from build123d import *

# Parameters (mm, degrees)
F0_R     = 4.05
F1_DEPTH = 20
F2_DEPTH = 17
F3_R     = 3
F4_R     = 4.05
F5_DEPTH = 219.9
F6_START = 103.2
F6_DEPTH = 43.7
F7_DEPTH = 8


with BuildPart() as f1:
    # F0 (on Top) → F1 (new body)
    with BuildSketch(Plane.XY):
        with BuildLine():
            Line((80, 54.9215728753), (80, 47.75))
            Line((80, 47.75), (100, 20))
            Line((100, 20), (100, 0))
            Line((100, 0), (100, -20))
            Line((100, -20), (80, -47.75))
            Line((80, -47.75), (80, -63.952777299))
            Line((80, -63.952777299), (92, -65))
            Line((92, -65), (112, -64.6363035163))
            Line((112, -64.6363035163), (112, 0))
            Line((112, 0), (112, 64.1046091914))
            Line((112, 64.1046091914), (81.7398235416, 64.1046091914))
            Line((81.7398235416, 64.1046091914), (80, 63.952777299))
            Line((80, 63.952777299), (80, 60.5784271247))
            ThreePointArc((80, 60.5784271247), (80.4926940638, 60.706795679), (81, 60.75))
            Line((81, 60.75), (89, 60.75))
            Line((89, 60.75), (95, 60.75))
            Line((95, 60.75), (105, 60.75))
            ThreePointArc((105, 60.75), (107.1213203436, 59.8713203436), (108, 57.75))
            ThreePointArc((108, 57.75), (107.1213203436, 55.6286796564), (105, 54.75))
            Line((105, 54.75), (95, 54.75))
            Line((95, 54.75), (89, 54.75))
            Line((89, 54.75), (81, 54.75))
            ThreePointArc((81, 54.75), (80.4926940638, 54.793204321), (80, 54.9215728753))
        make_face()
        with Locations((92, -47.75)):
            Circle(F0_R, mode=Mode.SUBTRACT)
        with Locations((92, 47.75)):
            Circle(F0_R, mode=Mode.SUBTRACT)
        Polygon((80, -63.952777299), (80, -47.75), (74.5151937008, -55.3601687402), (74.5151937008, -63.4741261601), align=None)
        with BuildLine():
            Line((74.5151937008, 55.3601687402), (80, 47.75))
            Line((80, 47.75), (80, 54.9215728753))
            ThreePointArc((80, 54.9215728753), (78, 57.75), (80, 60.5784271247))
            Line((80, 60.5784271247), (80, 63.952777299))
            Line((80, 63.952777299), (74.5151937008, 63.4741261601))
            Line((74.5151937008, 63.4741261601), (74.5151937008, 55.3601687402))
        make_face()
    extrude(amount=F1_DEPTH)

    # F0 (on Top) → F2 (join)
    with BuildSketch(Plane.XY):
        with BuildLine():
            ThreePointArc((105, 60.75), (102, 57.75), (105, 54.75))
            ThreePointArc((105, 54.75), (107.1213203436, 55.6286796564), (108, 57.75))
            ThreePointArc((108, 57.75), (107.1213203436, 59.8713203436), (105, 60.75))
        make_face()
        with BuildLine():
            Line((80, 60.5784271247), (80, 54.9215728753))
            ThreePointArc((80, 54.9215728753), (80.4926940638, 54.793204321), (81, 54.75))
            ThreePointArc((81, 54.75), (83.1213203436, 55.6286796564), (84, 57.75))
            ThreePointArc((84, 57.75), (83.1213203436, 59.8713203436), (81, 60.75))
            ThreePointArc((81, 60.75), (80.4926940638, 60.706795679), (80, 60.5784271247))
        make_face()
        with BuildLine():
            ThreePointArc((80, 60.5784271247), (78, 57.75), (80, 54.9215728753))
            Line((80, 54.9215728753), (80, 60.5784271247))
        make_face()
        with BuildLine():
            ThreePointArc((84, 57.75), (83.1213203436, 55.6286796564), (81, 54.75))
            Line((81, 54.75), (89, 54.75))
            ThreePointArc((89, 54.75), (86, 57.75), (89, 60.75))
            Line((89, 60.75), (81, 60.75))
            ThreePointArc((81, 60.75), (83.1213203436, 59.8713203436), (84, 57.75))
        make_face()
        with BuildLine():
            ThreePointArc((98, 57.75), (97.1213203436, 55.6286796564), (95, 54.75))
            Line((95, 54.75), (105, 54.75))
            ThreePointArc((105, 54.75), (102, 57.75), (105, 60.75))
            Line((105, 60.75), (95, 60.75))
            ThreePointArc((95, 60.75), (97.1213203436, 59.8713203436), (98, 57.75))
        make_face()
    extrude(amount=F2_DEPTH)

    # F3
    f3_edges = [f1.edges().sort_by_distance(p)[0] for p in [
        (74.515194, -55.360169, 10),
        (74.515194, -63.474126, 10),
        (100, -20, 10),
        (100, 20, 10),
        (74.515194, 55.360169, 10),
        (74.515194, 63.474126, 10),
    ]]
    fillet(f3_edges, radius=F3_R)

    # F4 (on Right) → F5 (cut)
    with BuildSketch(Plane.YZ):
        with Locations((0, 10)):
            Circle(F4_R)
    extrude(amount=F5_DEPTH, mode=Mode.SUBTRACT)

    # F4 (on Right) → F6 (cut)
    with BuildSketch(Plane.YZ.offset(F6_START)):
        Polygon((-3.7527767497, 3.5), (3.7527767497, 3.5), (7.5055534995, 10), (3.7527767497, 16.5), (-3.7527767497, 16.5), (-7.5055534995, 10), align=None)
        with Locations((0, 10)):
            Circle(F4_R, mode=Mode.SUBTRACT)
    extrude(amount=F6_DEPTH, mode=Mode.SUBTRACT)

    # F0 (on Top) → F7 (join)
    with BuildSketch(Plane.XY):
        with BuildLine():
            ThreePointArc((89, 60.75), (86, 57.75), (89, 54.75))
            ThreePointArc((89, 54.75), (91.1213203436, 55.6286796564), (92, 57.75))
            ThreePointArc((92, 57.75), (91.1213203436, 59.8713203436), (89, 60.75))
        make_face()
        with BuildLine():
            Line((95, 60.75), (89, 60.75))
            ThreePointArc((89, 60.75), (91.1213203436, 59.8713203436), (92, 57.75))
            ThreePointArc((92, 57.75), (92.8786796564, 59.8713203436), (95, 60.75))
        make_face()
        with BuildLine():
            ThreePointArc((92, 57.75), (92.8786796564, 55.6286796564), (95, 54.75))
            ThreePointArc((95, 54.75), (97.1213203436, 55.6286796564), (98, 57.75))
            ThreePointArc((98, 57.75), (97.1213203436, 59.8713203436), (95, 60.75))
            ThreePointArc((95, 60.75), (92.8786796564, 59.8713203436), (92, 57.75))
        make_face()
        with BuildLine():
            ThreePointArc((92, 57.75), (91.1213203436, 55.6286796564), (89, 54.75))
            Line((89, 54.75), (95, 54.75))
            ThreePointArc((95, 54.75), (92.8786796564, 55.6286796564), (92, 57.75))
        make_face()
    extrude(amount=F7_DEPTH)


solid = f1.part
Here's how the part is built. I have some questions about the finished solid (model axes, mm). A direction names the side the tool comes from. Coordinates: 2 decimals unless noted, no trailing zeros. Loops run counter-clockwise (first coordinate to the right, second up) from the corner with the lowest first, then second, coordinate; pieces in that order, holes last.
1. For P1, Ø4, axis at y = -2.5, z = 9, coming from the +X side; P2, Ø6, axis at y = -9.5, z = 12, coming from the -X side; P3, Ø1.5, axis at y = 38.5, z = 3.5, coming from the -X side; P4, Ø7.5, axis at x = 92, y = 47.75, coming from the +Z side, each with a flat end and sliding along its axis, tell me the tip position at first contact or that it passes through.
2. For faces 4 (the flat face through (100, 4.5, 9.9)), 5 (the cylindrical face through (95.86, 48.97, 9.86)), 6 (the flat face through (92, 58, 8)), 7 (the flat face through (97, 64.105, 10)), 8 (the flat face through (107.5, -5.6, 13.3)), which set-ups out of +Z, -Z, +X, -X, +Y, -Y let a thin tool reach every point of the face, with its end or its side?
3. Imagine slicing it at C-C, the plane z = 11.5. Count the separate pieces of the cut face and the enclosed holes in it, and give its area (3 significant figures).
4. Imagine slicing it at D-D, the plane y = 49. Please give me the cut outline in (x, z), and give its area (3 significant figures).
5. Imagine slicing it at A-A, the plane y = 0. Please give me the cut outline in (x, z), and give its area (3 significant figures).
6. I need wall thicknesses on L1, parallel to Y at x = 91, z = 10.25; L2, parallel to Z at x = 101.9, y = 0; L3, parallel to Y at x = 92, z = 8.75. Which ranges of each line are inside material? Lowest first, please.
7. If we mould it in two halves opening along X, with no side actions, what happens to faces 1 (the flat face through (74.515, -58, 10)), 2 (the flat face through (82, 58, 17)), 3 (the flat face through (107.5, 5.6, 6.7))? For each: pulls with the +X half, pulls with the -X half, needs draft (parallel to the pull), parting line crosses it, or undercut.
8. Imagine slicing it at B-B, the plane x = 84. Please give me the cut outline in (y, z), and give its area (3 significant figures).
Taken from the geometry:
1. P1: stops at x = 103.2
1. P2: stops at x = 100
1. P3: stops at x = 86.13
1. P4: passes through
2. face 4: +Z, -Z, -X
2. face 5: +Z, -Z
2. face 6: +Z
2. face 7: +Z, -Z, +X, -X, +Y
2. face 8: +X
3. separate pieces: 2
3. enclosed holes: 3
3. area: 2,590 mm2
4. outline: (79.1, 0) - (88.15, 0) - (88.15, 20) - (79.1, 20) - close; (95.85, 0) - (112, 0) - (112, 20) - (95.85, 20) - close
4. area: 504 mm2
5. outline: (100, 0) - (112, 0) - (112, 3.5) - (103.2, 3.5) - (103.2, 5.95) - (100, 5.95) - close; (100, 14.05) - (103.2, 14.05) - (103.2, 16.5) - (112, 16.5) - (112, 20) - (100, 20) - close
5. area: 99.7 mm2
6. L1: y = -64.91 to -51.67, -43.83 to -32.49, 32.49 to 43.83, 51.67 to 54.75, 60.75 to 64.1
6. L2: z = 0 to 5.95, 14.05 to 20
6. L3: y = -65 to -51.8, -43.7 to -31.1, 31.1 to 43.7, 51.8 to 54.75, 60.75 to 64.1
7. face 1: pulls with the -X half
7. face 2: undercut
7. face 3: needs draft
8. outline: (-64.3, 0) - (-42.2, 0) - (-42.2, 20) - (-64.3, 20) - close; (42.2, 0) - (64.1, 0) - (64.1, 20) - (60.75, 20) - (60.75, 17) - (54.75, 17) - (54.75, 20) - (42.2, 20) - close
8. area: 862 mm2
